from build123d import *

# Parameters (mm, degrees)
SKETCH1_W           = 12
SKETCH1_H           = 10
SKETCH1_W_2         = 4
SKETCH1_H_2         = 4
BOSS_EXTRUDE1_DEPTH = 4
SKETCH2_R           = 1.5
CUT_EXTRUDE1_DEPTH  = 12.532562595
CUT_EXTRUDE3_DEPTH  = 4


with BuildPart() as part:
    # Sketch1 → Boss-Extrude1 (new body)
    with BuildSketch(Plane(origin=(0, 0, 0), x_dir=(1, 0, 0), z_dir=(0, 1, 0))):
        Rectangle(SKETCH1_W, SKETCH1_H)
        with Locations((-4, -7)):
            Rectangle(SKETCH1_W_2, SKETCH1_H_2)
        with Locations((4, -7)):
            Rectangle(SKETCH1_W_2, SKETCH1_H_2)
    extrude(amount=BOSS_EXTRUDE1_DEPTH)

    # Sketch2 → Cut-Extrude1 (cut, through all)
    with BuildSketch(Plane(origin=(0, 4, 0), x_dir=(1, 0, 0), z_dir=(0, 1, 0))):
        with Locations(Location((-3, 1, 0), (0, 0, 270))):
            Circle(SKETCH2_R)
        with Locations(Location((3, 1, 0), (0, 0, 270))):
            Circle(SKETCH2_R)
    extrude(amount=-CUT_EXTRUDE1_DEPTH, mode=Mode.SUBTRACT)

    # Sketch3 → Cut-Extrude3 (cut)
    with BuildSketch(Plane(origin=(0, 4, 0), x_dir=(1, 0, 0), z_dir=(0, 1, 0))):
        with BuildLine():
            ThreePointArc((-6, 0), (-3.905124845, 3.586149799), (-1.9e-08, 5))
            Line((-1.9e-08, 5), (-6, 5))
            Line((-6, 5), (-6, 0))
        make_face()
        with BuildLine():
            ThreePointArc((-1.9e-08, 5), (3.905124831, 3.586149812), (6, 0))
            Line((6, 0), (6, 5))
            Line((6, 5), (-1.9e-08, 5))
        make_face()
    extrude(amount=-CUT_EXTRUDE3_DEPTH, mode=Mode.SUBTRACT)


solid = part.part
Model file for the job. Use its own axes, mm. A direction names the side the tool comes from. Give positions to 0.01 mm unless a question says otherwise; leave off trailing zeros. Write each loop counter-clockwise with the first axis right and the second up, starting at its lowest first coordinate (ties: lowest second). Pieces come first, ordered by that corner, then holes. Notation, with made-up numbers: M 30.25,5.5 L 48.25,5.5 A20 ccw 48.25,23.5 Z; hole C -28,54.5 d5. An arc over 180 degrees is marked long. One line per item, written item: value. Start each with the question number.
Q1. Saw through at D-D, the plane z = -1. Write the cut outline in (x, y), plus the area to 3 significant figures.
Q2. Saw through at B-B, the plane y = 1.65. Write the cut outline in (x, z).
Q3. Saw through at C-C, the plane x = 3. Write the cut outline in (y, z), plus the area to 3 significant figures.
Q4. Probe probe 1 along X at (y, z) = (3.4, 8); probe 2 along X at (y, z) = (3, -1); probe 3 along X at (y, z) = (3.8, -2). List the from-to ranges inside material, lowest first. Write a range as [from, to].
Q5. 3-axis set-ups, long thin cutter, end or side, ignore diameter. For faces 5 (the flat face through (-6, 2, 4)), 6 (the flat face through (0, 2, 5)): which of +Z, -Z, +X, -X, +Y, -Y reach the whole face in a straight line?
Q6. Saw through at A-A, the plane z = 8.25. Write the cut outline in (x, y), plus the area to 3 significant figures.
Q7. Two-plate mould, pull along Z, no slides. Class faces 1 (the cylindrical face through (1.536, 2.028, -1.325)), 2 (the flat face through (-2, 2, 7)), 3 (the flat face through (-4, 2, 9)), 4 (the cylindrical face through (-1.513, 2.028, -1.195)): +Z half, -Z half, draft (parallel to the pull), parting line (faces both ways), or undercut.
Q8. Drop flat-ended pins along their axis: pin 1 Ø2.5 at (x, z) = (3, -1) entering from +Y; pin 2 Ø2 at (x, y) = (0, 2.5) entering from +Z. Give the stop position or say it passes through.
Output values:
1. outline: M -5.73,0 L -4.5,0 L -4.5,4 L -5.73,4 Z; M -1.5,0 L 1.5,0 L 1.5,4 L -1.5,4 Z; M 4.5,0 L 5.73,0 L 5.73,4 L 4.5,4 Z
1. area: 21.8 mm²
2. outline: M -6,0 A6.1 ccw 6,0 L 6,9 L 2,9 L 2,5 L -2,5 L -2,9 L -6,9 Z; hole C -3,-1 d3; hole C 3,-1 d3
3. outline: M 0,-4.21 L 4,-4.21 L 4,-2.5 L 0,-2.5 Z; M 0,0.5 L 4,0.5 L 4,9 L 0,9 Z
3. area: 40.8 mm²
4. probe 1: x = [-6, -2], [2, 6]
4. probe 2: x = [-5.73, -4.5], [-1.5, 1.5], [4.5, 5.73]
4. probe 3: x = [-5.25, -4.12], [-1.88, 1.88], [4.12, 5.25]
5. face 5: +Z, -Z, -X, +Y, -Y
5. face 6: +Z, +Y, -Y
6. outline: M -6,0 L -2,0 L -2,4 L -6,4 Z; M 2,0 L 6,0 L 6,4 L 2,4 Z
6. area: 32.0 mm²
7. face 1: undercut
7. face 2: draft
7. face 3: +Z half
7. face 4: undercut
8. pin 1: passes through
8. pin 2: stops at z = 5
